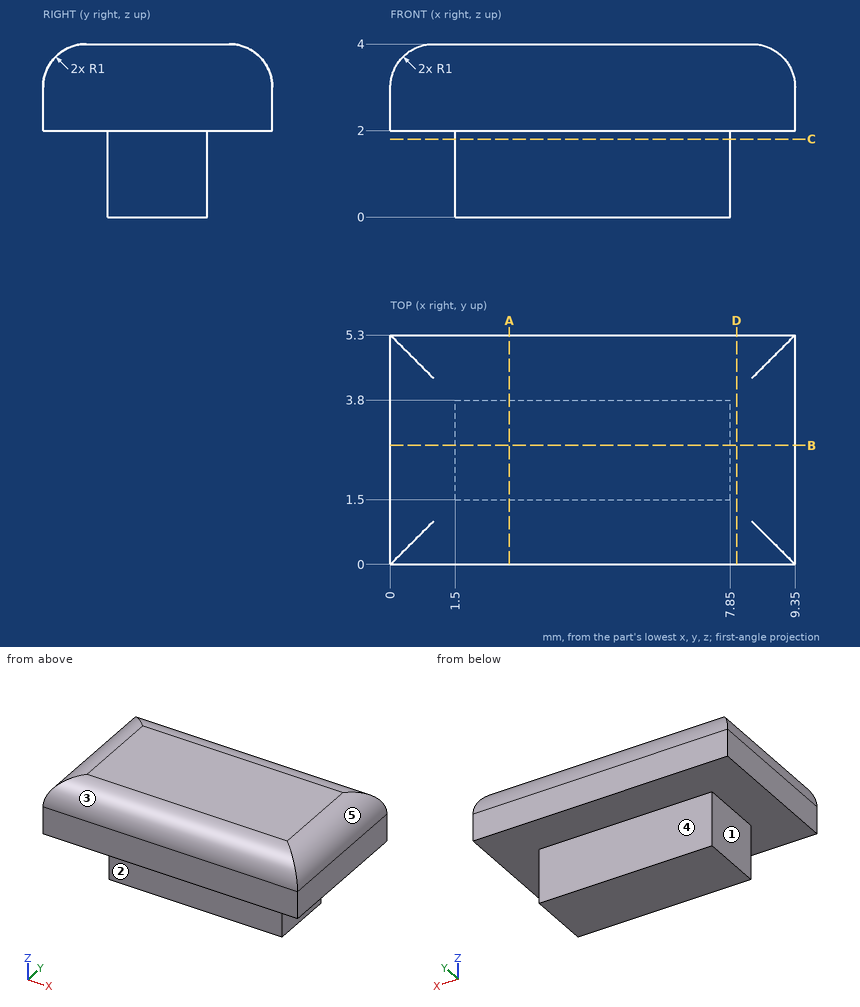
Drawing for the job (mm, zero at the part's lowest x, y, z). A direction names the side the tool comes from. Round coordinates to 2 decimals unless told otherwise and drop trailing zeros. Write each loop counter-clockwise with the first axis right and the second up, starting at its lowest first coordinate (ties: lowest second). Pieces come first, ordered by that corner, then holes. Notation, with made-up numbers: (-23.75, 55.5) - (10.25, 55.5) arc R11 ccw to (10.25, 63.5) - close; hole circle Ø7 at (-22.5, 37). An arc over 180 degrees is marked (long way). Write item = value, one per line. Start each with the question number.
Q1. Band-saw the part on D-D (x = 8). Give the cut face in (y, z).
Q2. Probe L1, parallel to X at y = 2.1, z = 1.3; L2, parallel to Z at x = 3.25, y = 4.2; L3, parallel to Y at x = 5.25, z = 0.4. List the from-to ranges inside material, lowest first. Write a range as from..to.
Q3. Which spindle directions (+Z, -Z, +X, -X, +Y, -Y) get a long thin tool onto all of the face, cutting with end or side? Do the marked faces 1, 2, 3, 4 and 5. Say none if no direction does.
Q4. Band-saw the part on C-C (z = 1.8). Give the cut face in (x, y).
Q5. Drop flat-ended pins along their axis: pin 1 (0.6 mm diameter, centred on x = 6, z = 0.5, fed in from +Y); pin 2 (1.6 mm diameter, centred on x = 3.5, z = 1, fed in from -Y); pin 3 (1.6 mm diameter, centred on y = 3, z = 1, fed in from -X). Give the stop position or say it passes through.
Q6. Band-saw the part on B-B (y = 2.75). Give the cut face in (x, z).
Q7. Band-saw the part on A-A (x = 2.75). Give the cut face in (y, z), then the cut area to 3 significant figures.
Answers below:
q1.outline = (0, 2) - (5.3, 2) - (5.3, 3) arc R1 ccw to (4.3, 4) - (1, 4) arc R1 ccw to (0, 3) - close
q2.L1 = 1.5..7.85
q2.L2 = 2..4
q2.L3 = 1.5..3.8
q3.face_1 = -Z, -X, +Y, -Y
q3.face_2 = -Z, +X, -X, -Y
q3.face_3 = +Z, +X, -X, -Y
q3.face_4 = -Z, +X, -X, +Y
q3.face_5 = +Z, +X, +Y, -Y
q4.outline = (1.5, 1.5) - (7.85, 1.5) - (7.85, 3.8) - (1.5, 3.8) - close
q5.pin_1 = 3.8
q5.pin_2 = 1.5
q5.pin_3 = 1.5
q6.outline = (0, 2) - (1.5, 2) - (1.5, 0) - (7.85, 0) - (7.85, 2) - (9.35, 2) - (9.35, 3) arc R1 ccw to (8.35, 4) - (1, 4) arc R1 ccw to (0, 3) - close
q7.outline = (0, 2) - (1.5, 2) - (1.5, 0) - (3.8, 0) - (3.8, 2) - (5.3, 2) - (5.3, 3) arc R1 ccw to (4.3, 4) - (1, 4) arc R1 ccw to (0, 3) - close
q7.area = 14.8 mm2
